```python
from build123d import *

# Parameters (mm, degrees)
F0_R     = 7
F1_DEPTH = 21.5


with BuildPart() as f1:
    # F0 (on Front) → F1 (new body, symmetric)
    with BuildSketch(Plane.XZ):
        with BuildLine():
            Line((67, 19), (62, 24))
            Line((62, 24), (38, 24))
            ThreePointArc((38, 24), (29.574973, 16.276069), (18.243085, 14.783252))
            Line((18.243085, 14.783252), (0, 18))
            Line((0, 18), (-7, 18))
            Line((-7, 18), (-14, 11))
            Line((-14, 11), (-14, -7))
            Line((-14, -7), (-7, -14))
            Line((-7, -14), (21.066626, -14))
            ThreePointArc((21.066626, -14), (24.331862, -15.213414), (26.012265, -18.264706))
            ThreePointArc((26.012265, -18.264706), (28.349095, -26.115672), (32.788067, -33))
            Line((32.788067, -33), (38, -33))
            Line((38, -33), (67, 0))
            Line((67, 0), (67, 19))
        make_face()
        Circle(F0_R, mode=Mode.SUBTRACT)
    extrude(amount=F1_DEPTH, both=True)


solid = f1.part
```
Model file for the job. Use its own axes, mm. A direction names the side the tool comes from. Give positions to 0.01 mm unless a question says otherwise; leave off trailing zeros. Order: outer loops, then holes, each group sorted by start corner. A loop starts at its lowest first (then second) coordinate and runs counter-clockwise, first axis right, second up.
1) Saw through at C-C, the plane z = 3.5. Write the cut outline in (x, y).
2) Pin check, flat tips, straight feed: pin 1 (2 mm diameter, centred on x = 24.5, y = -0.5, fed in from +Z); pin 2 (16 mm diameter, centred on x = 0, z = 0, fed in from +Y); pin 3 (2 mm diameter, centred on y = 5.5, z = -20.5, fed in from +X); pin 4 (10 mm diameter, centred on y = 4, z = -23, fed in from -X). Stop position of each tip, or through.
3) Wall check: probe 1 along Z at (x, y) = (0, -6); probe 2 along X at (y, z) = (6, 2.5); probe 3 along X at (y, z) = (3.5, -16). Give the ranges that are in metal, low to high.
4) 3-axis set-ups, long thin cutter, end or side, ignore diameter. For faces 1 (the flat face through (9.25, -0.3, 16.37)), 2 (the flat face through (7, 0, -14)), 3 (the flat face through (-3, 0, 18)): which of +Z, -Z, +X, -X, +Y, -Y reach the whole face in a straight line?
5) Saw through at A-A, the plane y = 5.5. Write the cut outline in (x, z), then the cut area to 3 significant figures.
6) Saw through at D-D, the plane x = 52. Write the cut outline in (y, z).
7) Saw through at B-B, the plane x = 1. Write the cut outline in (y, z).
Computed:
1. outline: (-14, -21.5) - (-6.06, -21.5) - (-6.06, 21.5) - (-14, 21.5) - close; (6.06, -21.5) - (67, -21.5) - (67, 21.5) - (6.06, 21.5) - close
2. pin 1: stops at z = 14.91
2. pin 2: stops at y = 21.5
2. pin 3: stops at x = 49.86
2. pin 4: stops at x = 25.97
3. probe 1: z = -14 to -7, 7 to 18
3. probe 2: x = -14 to -6.54, 6.54 to 67
3. probe 3: x = 25.07 to 52.94
4. face 1: +Z, +Y, -Y
4. face 2: -Z, -X, +Y, -Y
4. face 3: +Z, -X, +Y, -Y
5. outline: (-14, -7) - (-7, -14) - (21.07, -14) arc R5 cw to (26.01, -18.26) arc R29 ccw to (32.79, -33) - (38, -33) - (67, 0) - (67, 19) - (62, 24) - (38, 24) arc R19 cw to (18.24, 14.78) - (0, 18) - (-7, 18) - (-14, 11) - close; hole circle Ø14 at (0, 0)
5. area: 2,770 mm2
6. outline: (-21.5, -17.07) - (21.5, -17.07) - (21.5, 24) - (-21.5, 24) - close
7. outline: (-21.5, -14) - (21.5, -14) - (21.5, -6.93) - (-21.5, -6.93) - close; (-21.5, 6.93) - (21.5, 6.93) - (21.5, 17.82) - (-21.5, 17.82) - close
